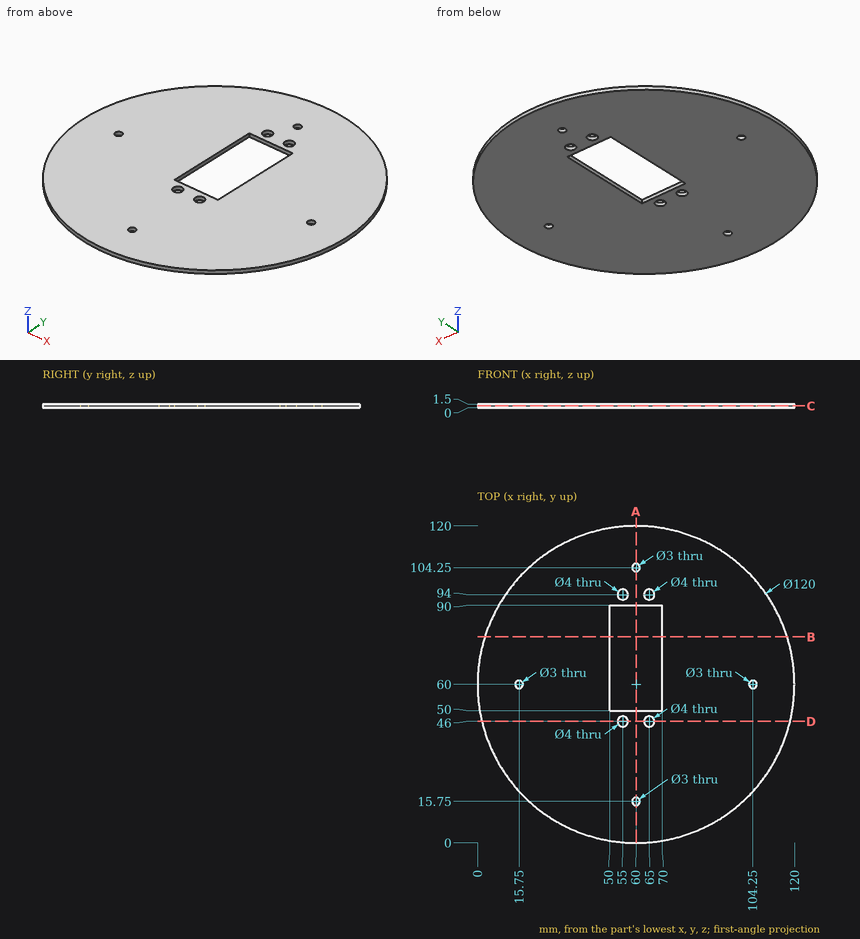
Design review of the part shown in the three views and the two pictorial views. Dimensions are in mm from the part's minimum x, y and z. Round coordinates to 2 decimals unless told otherwise and drop trailing zeros. Loops run counter-clockwise (first coordinate to the right, second up) from the corner with the lowest first, then second, coordinate; pieces in that order, holes last.
(1) We need section A-A (x = 60). Give the boundary of the cut face in (y, z).
Returned:
outline: (0, 0) - (14.25, 0) - (14.25, 1.5) - (0, 1.5) - close; (17.25, 0) - (50, 0) - (50, 1.5) - (17.25, 1.5) - close; (90, 0) - (102.75, 0) - (102.75, 1.5) - (90, 1.5) - close; (105.75, 0) - (120, 0) - (120, 1.5) - (105.75, 1.5) - close
(2) We need section C-C (z = 0.75). State how many separate pieces and enclosed holes the cut face has, plus the area to 3 significant figures.
Returned:
separate pieces: 1
enclosed holes: 9
area: 10,400 mm2
(3) Wall thickness on line 1 along Y through (x, z) = (60, 0.45); line 2 along Y through (x, z) = (55, 1.05); line 3 along Y through (x, z) = (15.75, 0.6): over which ranges is each line inside the solid? List them lowest first.
Returned:
line 1: y = 0 to 14.25, 17.25 to 50, 90 to 102.75, 105.75 to 120
line 2: y = 0.21 to 44, 48 to 50, 90 to 92, 96 to 119.79
line 3: y = 19.48 to 58.5, 61.5 to 100.52
(4) We need section D-D (y = 46). Give the boundary of the cut face in (x, z), plus the area to 3 significant figures.
Returned:
outline: (1.66, 0) - (53, 0) - (53, 1.5) - (1.66, 1.5) - close; (57, 0) - (63, 0) - (63, 1.5) - (57, 1.5) - close; (67, 0) - (118.34, 0) - (118.34, 1.5) - (67, 1.5) - close
area: 163 mm2
(5) We need section B-B (y = 78). Give the boundary of the cut face in (x, z), plus the area to 3 significant figures.
Returned:
outline: (2.76, 0) - (50, 0) - (50, 1.5) - (2.76, 1.5) - close; (70, 0) - (117.24, 0) - (117.24, 1.5) - (70, 1.5) - close
area: 142 mm2
